Part model, mm, in its own coordinate system. Round coordinates to 2 decimals unless told otherwise and drop trailing zeros. Loops run counter-clockwise (first coordinate to the right, second up) from the corner with the lowest first, then second, coordinate; pieces in that order, holes last. Notation, with made-up numbers: (-1.75, 85.5) - (31.25, 85.5) arc R17 ccw to (31.25, 91.5) - close; hole circle Ø3 at (23.25, 32.5). An arc over 180 degrees is marked (long way). Write each question's results on one line, items separated by ' | '. Start each with the question number.
(1) Cut at B-B, the plane z = -12.75. List the corners of the cut face in (x, y).
(2) Flat gauge pin, fed straight in: P1, Ø6, axis at x = -45, y = 0, coming from the -Z side. Where does the tip first touch, or does it go through?
(3) Cut at A-A, the plane x = -45. List the corners of the cut face in (y, z), then the cut area to 3 significant figures.
(4) Mould opens along X. For faces 1 (the face through (-1, 0, -20)), 2 (the face through (50, 0, -10)), 3 (the face through (-60, 0, -10)) say: released by +X, released by -X, zero draft, split by the parting line, or undercut.
(5) Cut at C-C, the plane y = 0. List the corners of the cut face in (x, z), then the cut area to 3 significant figures.
(6) Drill centre lines: L1, parallel to X at y = -0.25, z = -1; L2, parallel to Y at x = 45, z = -14.5; L3, parallel to X at y = 2, z = -7. Where is each one in solid material? Low to high.
from build123d import *

# Parameters (mm, degrees)
F0_W     = 120
F0_H     = 16
F1_DEPTH = 20
F3_D     = 10
F4_SIZE  = 0.2


with BuildPart() as f1:
    # F0 (on Top) → F1 (new body)
    with BuildSketch(Plane.XY):
        Rectangle(F0_W, F0_H)
    extrude(amount=-F1_DEPTH)

    # F3 (through all)
    with Locations(Plane.XY):
        with Locations((-45, 0), (45, 0)):
            Hole(F3_D / 2)

    # F4
    f4_edges = [f1.edges().sort_by_distance(p)[0] for p in [
        (0, 8, 0),
        (60, 0, 0),
        (-60, 0, 0),
        (0, -8, 0),
        (-50, 0, 0),
        (40, 0, 0),
        (-60, 8, -10),
        (-60, -8, -10),
        (-60, 0, -20),
        (0, 8, -20),
        (60, 0, -20),
        (0, -8, -20),
        (-50, 0, -20),
        (40, 0, -20),
        (60, 8, -10),
        (60, -8, -10),
    ]]
    chamfer(f4_edges, length=F4_SIZE)


solid = f1.part
A:
1) outline: (-60, -7.8) - (-59.8, -8) - (59.8, -8) - (60, -7.8) - (60, 7.8) - (59.8, 8) - (-59.8, 8) - (-60, 7.8) - close; hole circle Ø10 at (-45, 0); hole circle Ø10 at (45, 0)
2) P1: through
3) outline: (-8, -19.8) - (-7.8, -20) - (-5.2, -20) - (-5, -19.8) - (-5, -0.2) - (-5.2, 0) - (-7.8, 0) - (-8, -0.2) - close; (5, -19.8) - (5.2, -20) - (7.8, -20) - (8, -19.8) - (8, -0.2) - (7.8, 0) - (5.2, 0) - (5, -0.2) - close | area: 120 mm2
4) face 1: zero draft | face 2: undercut | face 3: released by -X
5) outline: (-60, -19.8) - (-59.8, -20) - (-50.2, -20) - (-50, -19.8) - (-50, -0.2) - (-50.2, 0) - (-59.8, 0) - (-60, -0.2) - close; (-40, -19.8) - (-39.8, -20) - (39.8, -20) - (40, -19.8) - (40, -0.2) - (39.8, 0) - (-39.8, 0) - (-40, -0.2) - close; (50, -19.8) - (50.2, -20) - (59.8, -20) - (60, -19.8) - (60, -0.2) - (59.8, 0) - (50.2, 0) - (50, -0.2) - close | area: 2,000 mm2
6) L1: -60 to -49.99, -40.01 to 40.01, 49.99 to 60 | L2: -8 to -5, 5 to 8 | L3: -60 to -49.58, -40.42 to 40.42, 49.58 to 60
